Geometry: final body of the model. Coordinates: model frame, mm. A direction names the side the tool comes from. Coordinates: 2 decimals unless noted, no trailing zeros. Loops run counter-clockwise (first coordinate to the right, second up) from the corner with the lowest first, then second, coordinate; pieces in that order, holes last. Notation, with made-up numbers: (14, 43) -> (27, 43) arc R6 ccw to (27, 54) -> close; hole circle Ø1 at (54.25, 45.25). An arc over 180 degrees is marked (long way). One line per item, written item: value. Start each with the question number.
Item 1: Mould query, pull axis Y, two halves, no side actions, for faces 4 (the flat face through (-30, 30, 0)), 5 (the cylindrical face through (47.69, 15.02, 9.39)), 6 (the flat face through (-1, 1, 12.7)). Classes: +Y half, -Y half, draft (parallel to the pull), parting line (faces both ways), or undercut.
Item 2: Ray query, probe 1 along Y at (x, z) = (0, 3.5); probe 2 along Z at (x, y) = (38, -21); probe 3 along Z at (x, y) = (-27, 26). Return the intervals inside material, ascending. Write a range as from..to.
Item 3: Section query C-C on x = 21. Return loops of the section in (y, z), then the cut area to 3 significant figures.
Item 4: Section query D-D on z = 16. Return loops of the section in (x, y), then the cut area to 3 significant figures.
Item 5: Section query B-B on y = 7. Return loops of the section in (x, z).
Item 6: Section query A-A on z = 10.5. Return loops of the section in (x, y).
Item 7: Contact query for flat-ended pins moving along their axis: pin 1 Ø2.5 at (x, z) = (44, 1.5) entering from +Y; pin 2 Ø3 at (x, z) = (-4.5, 8.5) entering from -Y; pin 3 Ø3.5 at (y, z) = (43, 2) entering from +X. Output: stop coordinate, or through.
Item 8: Set-up query: faces 1 (the flat face through (-1, 1, 19.05)), 2 (the cylindrical face through (-30.023, 29.37, 1.479)), 3 (the flat face through (29, -31, 3)). Return all of +Z, -Z, +X, -X, +Y, -Y with unobstructed straight access to the full face (end or side cutting, diameter ignored); none if empty.
from build123d import *

# Parameters (mm, degrees)
F3_DEPTH = 3
F2_R     = 50
F4_DEPTH = 12.7
F5_R     = 50
F5_R_2   = 45
F6_DEPTH = 6.35


with BuildPart() as f3:
    # F2 (on Top) → F3 (new body)
    with BuildSketch(Plane.XY):
        with BuildLine():
            Line((0, 42), (0, 45))
            ThreePointArc((0, 45), (-31.8198051534, 31.8198051534), (-45, 0))
            Line((-45, 0), (-42, 0))
            ThreePointArc((-42, 0), (-29.6984848098, 29.6984848098), (0, 42))
        make_face()
    extrude(amount=F3_DEPTH)



with BuildPart() as f3b:
    # F2 (on Top) → F3, piece 2 (new body)
    with BuildSketch(Plane.XY):
        with BuildLine():
            ThreePointArc((0, -45), (31.8198051534, -31.8198051534), (45, 0))
            Line((45, 0), (42, 0))
            ThreePointArc((42, 0), (29.6984848098, -29.6984848098), (0, -42))
            Line((0, -42), (0, -45))
        make_face()
    extrude(amount=F3_DEPTH)


with BuildPart() as f3_1:
    add(f3.part)

    add(f3b.part)  # F4 merges F3b
    # F2 (on Top) → F4 (join)
    with BuildSketch(Plane.XY):
        Circle(F2_R)
        with BuildLine():
            ThreePointArc((0, 45), (31.8198051534, 31.8198051534), (45, 0))
            ThreePointArc((45, 0), (31.8198051534, -31.8198051534), (0, -45))
            ThreePointArc((0, -45), (-31.8198051534, -31.8198051534), (-45, 0))
            ThreePointArc((-45, 0), (-31.8198051534, 31.8198051534), (0, 45))
        make_face(mode=Mode.SUBTRACT)
    extrude(amount=F4_DEPTH)

    # F5 (on face) → F6 (join)
    with BuildSketch(Plane.XY.offset(12.7)):
        Circle(F5_R)
        Circle(F5_R_2, mode=Mode.SUBTRACT)
        Circle(F5_R_2)
    extrude(amount=F6_DEPTH)


solid = f3_1.part
Reply:
1. face 4: draft
1. face 5: parting line
1. face 6: undercut
2. probe 1: y = -50..-45, 45..50
2. probe 2: z = 0..3, 12.7..19.05
2. probe 3: z = 12.7..19.05
3. outline: (-45.38, 0) -> (-36.37, 0) -> (-36.37, 3) -> (-39.8, 3) -> (-39.8, 12.7) -> (39.8, 12.7) -> (39.8, 0) -> (45.38, 0) -> (45.38, 19.05) -> (-45.38, 19.05) -> close
3. area: 728 mm²
4. outline: circle Ø100 at (0, 0)
4. area: 7,850 mm²
5. outline: (-49.51, 0) -> (-41.41, 0) -> (-41.41, 3) -> (-44.45, 3) -> (-44.45, 12.7) -> (44.45, 12.7) -> (44.45, 0) -> (49.51, 0) -> (49.51, 19.05) -> (-49.51, 19.05) -> close
6. outline: circle Ø100 at (0, 0); hole circle Ø90 at (0, 0)
7. pin 1: stops at y = 25.93
7. pin 2: stops at y = -49.91
7. pin 3: stops at x = 28.26
8. face 1: +Z, +X, -X, +Y, -Y
8. face 2: -Z
8. face 3: none
